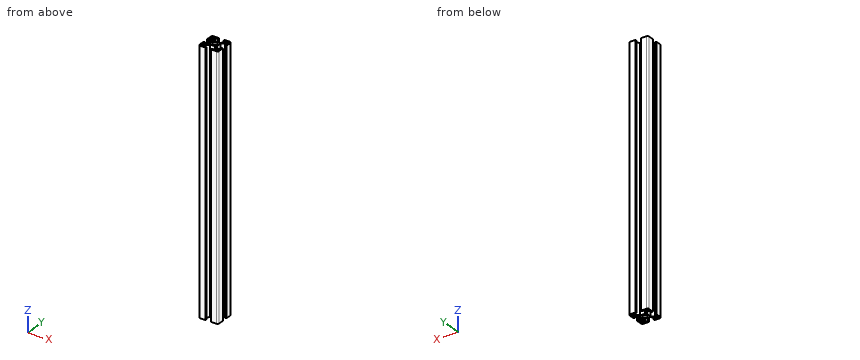
Autodesk Inventor part; units mm, degrees
ref_plane "YZ Plane" through (0, 0, 0) normal (1, 0, 0) x (0, 1, 0)
ref_plane "XZ Plane" through (0, 0, 0) normal (0, 1, 0) x (-1, 0, 0)
ref_plane "XY Plane" through (0, 0, 0) normal (0, 0, 1) x (1, 0, 0)
sketch "Sketch1" plane through (0, 0, 0) normal (0, 0, 1) x (1, 0, 0)
  circle A0 centre (-11.375, 11.375) radius 2.1
  circle A1 centre (-11.375, -11.375) radius 2.1
  line L0 (-15, 4.1) -> (-12.9, 4.1)
  line L1 (-12.9, 4.1) -> (-12.9, 8.28)
  line L2 (-12.9, 8.28) -> (-9.85, 8.28)
  line L3 (-9.85, 8.28) -> (-5.8, 4.23)
  line L4 (-5.8, 4.23) -> (-5.8, -4.23)
  line L5 (-5.8, -4.23) -> (-9.85, -8.28)
  line L6 (-9.85, -8.28) -> (-12.9, -8.28)
  line L7 (-12.9, -8.28) -> (-12.9, -4.1)
  line L8 (-12.9, -4.1) -> (-15, -4.1)
  line L9 (-15, -4.1) -> (-15, -13)
  arc A2 (-15, -13) -> (-13, -15) centre (-13, -13) ccw
  line L10 (-13, -15) -> (-4.1, -15)
  line L11 (-4.1, -15) -> (-4.1, -12.9)
  line L12 (-4.1, -12.9) -> (-8.28, -12.9)
  line L13 (-8.28, -12.9) -> (-8.28, -9.85)
  line L14 (-8.28, -9.85) -> (-3.719, -5.289)
  line L15 (-3.719, -5.289) -> (3.719, -5.289)
  line L16 (3.719, -5.289) -> (8.28, -9.85)
  line L17 (8.28, -9.85) -> (8.28, -12.9)
  line L18 (8.28, -12.9) -> (4.1, -12.9)
  line L19 (4.1, -12.9) -> (4.1, -15)
  line L20 (4.1, -15) -> (13, -15)
  arc A3 (13, -15) -> (15, -13) centre (13, -13) ccw
  line L21 (15, -13) -> (15, -4.1)
  line L22 (15, -4.1) -> (12.9, -4.1)
  line L23 (12.9, -4.1) -> (12.9, -8.28)
  line L24 (12.9, -8.28) -> (9.85, -8.28)
  line L25 (9.85, -8.28) -> (5.8, -4.23)
  line L26 (5.8, -4.23) -> (5.8, 4.23)
  line L27 (5.8, 4.23) -> (9.85, 8.28)
  line L28 (9.85, 8.28) -> (12.9, 8.28)
  line L29 (12.9, 8.28) -> (12.9, 4.1)
  line L30 (12.9, 4.1) -> (15, 4.1)
  line L31 (15, 4.1) -> (15, 13)
  arc A4 (15, 13) -> (13, 15) centre (13, 13) ccw
  line L32 (13, 15) -> (4.1, 15)
  line L33 (4.1, 15) -> (4.1, 12.9)
  line L34 (4.1, 12.9) -> (8.28, 12.9)
  line L35 (8.28, 12.9) -> (8.28, 9.85)
  line L36 (8.28, 9.85) -> (3.719, 5.289)
  line L37 (3.719, 5.289) -> (-3.719, 5.289)
  line L38 (-3.719, 5.289) -> (-8.28, 9.85)
  line L39 (-8.28, 9.85) -> (-8.28, 12.9)
  line L40 (-8.28, 12.9) -> (-4.1, 12.9)
  line L41 (-4.1, 12.9) -> (-4.1, 15)
  line L42 (-4.1, 15) -> (-13, 15)
  arc A5 (-13, 15) -> (-15, 13) centre (-13, 13) ccw
  line L43 (-15, 13) -> (-15, 4.1)
  circle A6 centre (0, 0) radius 3.4
  circle A7 centre (11.375, 11.375) radius 2.1
  circle A8 centre (11.375, -11.375) radius 2.1
extrude "Extrusion1" add sketch "Sketch1" against normal blind 400
properties part number "Metal Profile 40 cm" material "Aluminum 6061-AHC"
Design review of the part built by this model. Coordinates are the model's own, in mm. Round coordinates to 2 decimals unless told otherwise and drop trailing zeros. Write each loop counter-clockwise with the first axis right and the second up, starting at its lowest first coordinate (ties: lowest second). Pieces come first, ordered by that corner, then holes. Notation, with made-up numbers: (78.5, 6.5) - (118.5, 6.5) arc R15 ccw to (118.5, 24.5) - close; hole circle Ø11 at (62, 6). An arc over 180 degrees is marked (long way). Use a Markdown table: item, result. Add a question column.
1. Wall thickness on probe 1 along Y at (x, z) = (10, -67.5); probe 2 along Y at (x, z) = (9.75, -241.5); probe 3 along X at (y, z) = (-5.5, -33.5): over which ranges is each line inside the solid? List them lowest first.
2. We need section B-B (x = 0). State the section outline as (y, z) points.
3. We need section C-C (z = -265.5). Count the separate pieces of the cut face and the enclosed holes in it, then the cut area to 3 significant figures.
4. We need section A-A (y = 0). State the section outline as (x, z) points.
5. Clearance check with flat-ended pins moving along their axes: pin 1 (6 mm diameter, centred on x = 0, z = -171, fed in from +Y); pin 2 (0.6 mm diameter, centred on x = -14, z = -153.5, fed in from +Y); pin 3 (8 mm diameter, centred on x = 0, z = -191.5, fed in from +Y). State where each tip first meets the part, or that it passes through.
Output:
| question | item | result |
|---|---|---|
| 1 | probe 1 | y = -15 to -12.96, -9.79 to -8.28, 8.28 to 9.79, 12.96 to 15 |
| 1 | probe 2 | y = -15 to -12.71, -10.04 to -8.18, 8.18 to 10.04, 12.71 to 15 |
| 1 | probe 3 | x = -15 to -12.9, -7.07 to -3.93, 3.93 to 7.07, 12.9 to 15 |
| 2 | outline | (-5.29, -400) - (-3.4, -400) - (-3.4, 0) - (-5.29, 0) - close; (3.4, -400) - (5.29, -400) - (5.29, 0) - (3.4, 0) - close |
| 3 | separate pieces | 1 |
| 3 | enclosed holes | 5 |
| 3 | area | 323 mm2 |
| 4 | outline | (-5.8, -400) - (-3.4, -400) - (-3.4, 0) - (-5.8, 0) - close; (3.4, -400) - (5.8, -400) - (5.8, 0) - (3.4, 0) - close |
| 5 | pin 1 | stops at y = 5.29 |
| 5 | pin 2 | stops at y = 14.87 |
| 5 | pin 3 | stops at y = 5.57 |
